```python
from build123d import *

# Parameters (mm, degrees)
F0_W     = 100
F0_H     = 100
F1_DEPTH = 5
F3_DEPTH = 25
F4_R     = 2.1
F5_DEPTH = 25


with BuildPart() as f1:
    # F0 (on Top) → F1 (new body)
    with BuildSketch(Plane.XY):
        with Locations((50, 50)):
            Rectangle(F0_W, F0_H)
    extrude(amount=F1_DEPTH)

    # F2 (on face) → F3 (cut)
    with BuildSketch(Plane.XY.offset(5)):
        with BuildLine():
            Line((9.80931, 13.995452), (10.189486, 13.995509))
            ThreePointArc((10.189486, 13.995509), (9.999397, 14), (9.80931, 13.995452))
        make_face()
        with BuildLine():
            Line((39.999397, 14), (10.189486, 13.995509))
            Line((10.189486, 13.995509), (9.80931, 13.995452))
            ThreePointArc((9.80931, 13.995452), (6.001138, 9.9046), (10.000056, 6))
            Line((10.000056, 6), (39.942331, 6.000416))
            ThreePointArc((39.942331, 6.000416), (43.999898, 9.971466), (39.999397, 14))
        make_face()
        with BuildLine():
            Line((10.000056, 86), (39.942331, 86.000416))
            ThreePointArc((39.942331, 86.000416), (43.999898, 89.971466), (39.999397, 94))
            Line((39.999397, 94), (10.189486, 93.995509))
            Line((10.189486, 93.995509), (9.80931, 93.995452))
            ThreePointArc((9.80931, 93.995452), (6.001138, 89.9046), (10.000056, 86))
        make_face()
        with BuildLine():
            Line((9.80931, 93.995452), (10.189486, 93.995509))
            ThreePointArc((10.189486, 93.995509), (9.999397, 94), (9.80931, 93.995452))
        make_face()
        with BuildLine():
            Line((60.000056, 6), (89.942331, 6.000416))
            ThreePointArc((89.942331, 6.000416), (93.999898, 9.971466), (89.999397, 14))
            Line((89.999397, 14), (60.189486, 13.995509))
            Line((60.189486, 13.995509), (59.80931, 13.995452))
            ThreePointArc((59.80931, 13.995452), (56.001138, 9.9046), (60.000056, 6))
        make_face()
        with BuildLine():
            Line((59.80931, 13.995452), (60.189486, 13.995509))
            ThreePointArc((60.189486, 13.995509), (59.999397, 14), (59.80931, 13.995452))
        make_face()
        with BuildLine():
            Line((60.000056, 86), (89.942331, 86.000416))
            ThreePointArc((89.942331, 86.000416), (93.999898, 89.971466), (89.999397, 94))
            Line((89.999397, 94), (60.189486, 93.995509))
            Line((60.189486, 93.995509), (59.80931, 93.995452))
            ThreePointArc((59.80931, 93.995452), (56.001138, 89.9046), (60.000056, 86))
        make_face()
        with BuildLine():
            Line((59.80931, 93.995452), (60.189486, 93.995509))
            ThreePointArc((60.189486, 93.995509), (59.999397, 94), (59.80931, 93.995452))
        make_face()
    extrude(amount=-F3_DEPTH, mode=Mode.SUBTRACT)

    # F4 (on face) → F5 (cut)
    with BuildSketch(Plane.XY.offset(5)):
        with Locations((20, 73)):
            Circle(F4_R)
        with Locations((20, 27)):
            Circle(F4_R)
        with Locations((80, 27)):
            Circle(F4_R)
        with Locations((80, 73)):
            Circle(F4_R)
    extrude(amount=-F5_DEPTH, mode=Mode.SUBTRACT)


solid = f1.part
```
Input: part model. Units: mm. Frame: model coordinates. A direction names the side the tool comes from. Give positions to 0.01 mm unless a question says otherwise; leave off trailing zeros. Order: outer loops, then holes, each group sorted by start corner. A loop starts at its lowest first (then second) coordinate and runs counter-clockwise, first axis right, second up. Notation, with made-up numbers: M 30.25,17 L 34.25,17 A21 cw 34.25,34 Z; hole C -8.75,49 d9. An arc over 180 degrees is marked long. One line per question, with ' | ' between items.
1) Section C-C on x = 80. Output: boundary loops of the cut face in (y, z), and give its area (3 significant figures).
Filled in:
outline: M 0,0 L 6,0 L 6,5 L 0,5 Z; M 14,0 L 24.9,0 L 24.9,5 L 14,5 Z; M 29.1,0 L 70.9,0 L 70.9,5 L 29.1,5 Z; M 75.1,0 L 86,0 L 86,5 L 75.1,5 Z; M 94,0 L 100,0 L 100,5 L 94,5 Z | area: 378 mm2
2) Contact query for flat-ended pins moving along their axis: P1, Ø2.5, axis at x = 31, z = 2.5, coming from the -Y side; P2, Ø2.5, axis at x = 20, y = 27, coming from the -Z side. Output: stop coordinate, or through.
Filled in:
P1: stops at y = 0 | P2: passes through
3) Section A-A on y = 11. Output: boundary loops of the cut face in (x, z), and give its area (3 significant figures).
Filled in:
outline: M 0,0 L 6.13,0 L 6.13,5 L 0,5 Z; M 43.87,0 L 56.13,0 L 56.13,5 L 43.87,5 Z; M 93.87,0 L 100,0 L 100,5 L 93.87,5 Z | area: 123 mm2
4) Section B-B on z = 2.35. State how many separate pieces and enclosed holes the cut face has, and give its area (3 significant figures).
Filled in:
separate pieces: 1 | enclosed holes: 8 | area: 8,780 mm2
5) Access query for faces 1 (the face through (0, 49, 2)), 2 (the face through (6, 10, 3)). Directions: +Z, -Z, +X, -X, +Y, -Y. A direction counts if a zero-diameter tool reaches every point of the face in a straight line with its end or side. Return the directions, or none.
Filled in:
face 1: +Z, -Z, -X, +Y, -Y | face 2: +Z, -Z
6) Draft query along Y for faces 3 (the face through (49, 51, 0)), 4 (the face through (22.003, 27.631, 2.535)), 5 (the face through (49, 100, 2)). Return one class per face: pulls with the +Y half, pulls with the -Y half, needs draft (parallel to the pull), parting line crosses it, or undercut.
Filled in:
face 3: needs draft | face 4: undercut | face 5: pulls with the +Y half
7) Ray query, L1, parallel to Y at x = 20, z = 1.6; L2, parallel to Y at x = 74, z = 0.5; L3, parallel to X at y = 9.5, z = 1.8. Return the intervals inside material, ascending.
Filled in:
L1: y = 0 to 6, 14 to 24.9, 29.1 to 70.9, 75.1 to 86, 94 to 100 | L2: y = 0 to 6, 14 to 86, 94 to 100 | L3: x = 0 to 6.03, 43.97 to 56.03, 93.97 to 100
8) Section D-D on x = 66. Output: boundary loops of the cut face in (y, z).
Filled in:
outline: M 0,0 L 6,0 L 6,5 L 0,5 Z; M 14,0 L 86,0 L 86,5 L 14,5 Z; M 94,0 L 100,0 L 100,5 L 94,5 Z
